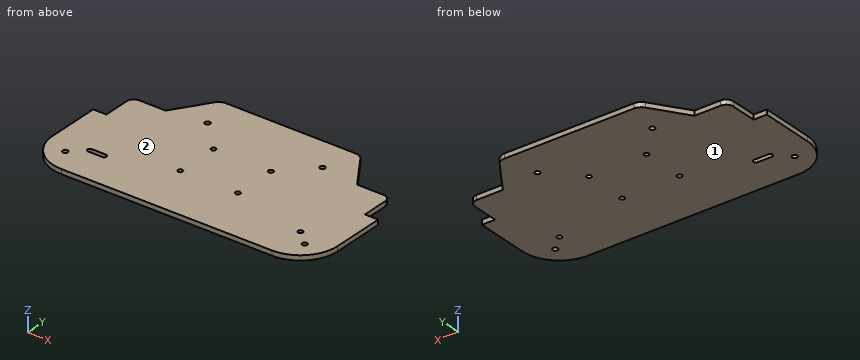
from build123d import *

# Parameters (mm, degrees)
SKETCH1_R           = 1.7145
SKETCH1_R_2         = 1.5875
BOSS_EXTRUDE1_DEPTH = 3.175
FILLET1_R           = 6.35


with BuildPart() as part:
    # Sketch1 → Boss-Extrude1 (new body)
    with BuildSketch(Plane.XY.offset(-196.85)):
        with BuildLine():
            Line((63.5, -114.3), (46.418820715, -88.9))
            Line((46.418820715, -88.9), (-46.418820715, -88.9))
            Line((-46.418820715, -88.9), (-63.5, -114.3))
            Line((-63.5, -114.3), (-80.9625, -114.3))
            ThreePointArc((-80.9625, -114.3), (-84.330096045, -115.694903955), (-85.725, -119.0625))
            Line((-85.725, -119.0625), (-85.725, -136.525))
            Line((-85.725, -136.525), (-94.488, -136.525))
            Line((-94.488, -136.525), (-94.488, -171.45))
            ThreePointArc((-94.488, -171.45), (-87.271696875, -188.871696875), (-69.85, -196.088))
            Line((-69.85, -196.088), (69.85, -196.088))
            ThreePointArc((69.85, -196.088), (87.271696875, -188.871696875), (94.488, -171.45))
            Line((94.488, -171.45), (94.488, -136.525))
            Line((94.488, -136.525), (85.725, -136.525))
            Line((85.725, -136.525), (85.725, -119.0625))
            ThreePointArc((85.725, -119.0625), (84.330096045, -115.694903955), (80.9625, -114.3))
            Line((80.9625, -114.3), (63.5, -114.3))
        make_face()
        with Locations((-79.375, -180.213)):
            Circle(SKETCH1_R, mode=Mode.SUBTRACT)
        with BuildLine():
            ThreePointArc((-69.85, -173.0375), (-71.4375, -171.45), (-69.85, -169.8625))
            Line((-69.85, -169.8625), (-60.325, -169.8625))
            ThreePointArc((-60.325, -169.8625), (-58.7375, -171.45), (-60.325, -173.0375))
            Line((-60.325, -173.0375), (-69.85, -173.0375))
        make_face(mode=Mode.SUBTRACT)
        with Locations((-19.05, -159.40600326)):
            Circle(SKETCH1_R_2, mode=Mode.SUBTRACT)
        with Locations((-19.05, -130.83100326)):
            Circle(SKETCH1_R_2, mode=Mode.SUBTRACT)
        with Locations((-38.1, -111.125)):
            Circle(SKETCH1_R, mode=Mode.SUBTRACT)
        with Locations((19.05, -159.40600326)):
            Circle(SKETCH1_R_2, mode=Mode.SUBTRACT)
        with Locations((79.375, -180.213)):
            Circle(SKETCH1_R, mode=Mode.SUBTRACT)
        with Locations((69.85, -171.45)):
            Circle(SKETCH1_R_2, mode=Mode.SUBTRACT)
        with Locations((19.05, -130.83100326)):
            Circle(SKETCH1_R_2, mode=Mode.SUBTRACT)
        with Locations((38.1, -111.125)):
            Circle(SKETCH1_R, mode=Mode.SUBTRACT)
    extrude(amount=-BOSS_EXTRUDE1_DEPTH)

    # Fillet1
    fillet1_edges = [part.edges().sort_by_distance(p)[0] for p in [
        (-46.418820715, -88.9, -198.4375),
        (46.418820715, -88.9, -198.4375),
    ]]
    fillet(fillet1_edges, radius=FILLET1_R)


solid = part.part
CAD build for the part. Positions are in the model's coordinates, mm. Face numbers are marked on the shaded views. Round coordinates to 2 decimals unless told otherwise and drop trailing zeros. Loops run counter-clockwise (first coordinate to the right, second up) from the corner with the lowest first, then second, coordinate; pieces in that order, holes last. Notation, with made-up numbers: (89, -1) - (122, -1) arc R21 ccw to (122, 34) - close; hole circle Ø9 at (79.5, 84.25). An arc over 180 degrees is marked (long way). Put each result on its own line as item: value.
1. Wall check: line 1 (Y direction, x = 19.05, z = -198.05); line 2 (X direction, y = -159.5, z = -199.6); line 3 (Y direction, x = 69.85, z = -197.7). Give the ranges that are in metal, low to high.
Geometry check:
line 1: -196.09 to -160.99, -157.82 to -132.42, -129.24 to -88.9
line 2: -94.49 to -20.63, -17.47 to 17.47, 20.63 to 94.49
line 3: -196.09 to -173.04, -169.86 to -114.3
2. Two-plate mould, pull along Z, no slides. Class the marked faces 1 and 2: released by +Z, released by -Z, zero draft, split by the parting line, or undercut.
Geometry check:
face 1: released by -Z
face 2: released by +Z
3. Slice it at B-B on y = -122. List the corners of the cut face in (x, z) (3 decimals), and give its area (3 significant figures).
Geometry check:
outline: (-85.725, -200.025) - (85.725, -200.025) - (85.725, -196.85) - (-85.725, -196.85) - close
area: 544 mm²
4. Slice it at C-C on x = 56. List the corners of the cut face in (y, z) (3 decimals).
Geometry check:
outline: (-196.088, -200.025) - (-103.147, -200.025) - (-103.147, -196.85) - (-196.088, -196.85) - close
5. Slice it at A-A on z = -197.6. Give the number of separate pieces and of enclosed holes in the cut face, and give its area (3 significant figures).
Geometry check:
separate pieces: 1
enclosed holes: 10
area: 17,500 mm²
6. Pin check, flat tips, straight feed: P1, Ø2.5, axis at x = 19.05, y = -130.83, coming from the -Z side; P2, Ø1.5, axis at y = -123, z = -197.5, coming from the -X side (3 decimals); P3, Ø1, axis at x = -90, z = -199, coming from the +Y side (3 decimals); P4, Ø1.6, axis at y = -131, z = -197.5, coming from the +X side (3 decimals). Stop position of each tip, or through.
Geometry check:
P1: through
P2: x = -85.725
P3: y = -136.525
P4: x = 85.725
